Autodesk Fusion 360 part; units mm, degrees
box "BoxPrimitive1" add length 20.5 width 45.5 height 1.5 placed x (0, 1, 0) y (-1, 0, 0) z (0, 0, 1) at (45.5, 0, 0)
sketch "Sketch2" plane through (0, 0, 1.5) normal (0, 0, 1) x (-1, 0, 0)
  line L0 (-45.5, -20.5) -> (0, -20.5)
  line L1 (0, -20.5) -> (0, 0)
  line L2 (0, 0) -> (-45.5, 0)
  line L3 (-45.5, 0) -> (-45.5, -20.5)
  line L4 (-45.5, -20.5) -> (-35.75, -20.5)
  line L5 (-35.75, -20.5) -> (-35.75, -10.25)
  line L6 (0, -20.5) -> (-9.75, -20.5)
  line L7 (-9.75, -20.5) -> (-9.75, -10.25)
  dimension "d6" = 9.75
  dimension "d7" = 10.25
  dimension "d10" = 9.75
  dimension "d11" = 10.25
cylinder "CylinderPrimitive1" add diameter 16 height 12 placed x (1, 0, 0) y (0, 1, 0) z (0, 0, 1) at (35.75, 10.25, 1.5)
cylinder "CylinderPrimitive2" add diameter 16 height 12 placed x (1, 0, 0) y (0, 1, 0) z (0, 0, 1) at (9.75, 10.25, 1.5)
Can you work these out from the model? Positions are in its coordinate system, mm. A direction names the side the tool comes from. Coordinates: 2 decimals unless noted, no trailing zeros. Order: outer loops, then holes, each group sorted by start corner. A loop starts at its lowest first (then second) coordinate and runs counter-clockwise, first axis right, second up. Notation, with made-up numbers: M 47,53.25 L 73,53.25 A20 ccw 73,71.25 Z; hole C 18.25,58 d4. An arc over 180 degrees is marked long. Answer as CSV lines item,"result".
(1) Suppose I cut it at A-A on x = 35.75. Please give me the cut outline in (y, z).
Geometry check:
outline,"M 0,0 L 20.5,0 L 20.5,1.5 L 18.25,1.5 L 18.25,13.5 L 2.25,13.5 L 2.25,1.5 L 0,1.5 Z"
(2) Suppose I cut it at D-D on x = 14. Please give me the cut outline in (y, z), plus the area to 3 significant figures.
Geometry check:
outline,"M 0,0 L 20.5,0 L 20.5,1.5 L 17.03,1.5 L 17.03,13.5 L 3.47,13.5 L 3.47,1.5 L 0,1.5 Z"
area,"193 mm^2"
(3) Please list where these lines run through material, in increasing order: L1, parallel to Z at x = 41.5, y = 17; L2, parallel to X at y = 3, z = 10.5; L3, parallel to X at y = 10, z = 10.75.
Geometry check:
L1,"0 to 1.5"
L2,"6.37 to 13.13, 32.37 to 39.13"
L3,"1.75 to 17.75, 27.75 to 43.75"
(4) I'm going to push flat-ended pins straight in: pin 1 (5 mm diameter, centred on x = 38, z = 10.5, fed in from +Y); pin 2 (2 mm diameter, centred on x = 14.5, z = 4.5, fed in from +Y); pin 3 (3 mm diameter, centred on x = 25, y = 3, fed in from +Z). Where does each tip first touch, or does it pass through?
Geometry check:
pin 1,"y = 18.25"
pin 2,"y = 17.32"
pin 3,"z = 1.5"
(5) If we mould it in two halves opening along X, with no side actions, what happens to faces 3 (the flat face through (22, 10, 1.5)), 4 (the flat face through (45.5, 10, 1)), 5 (the flat face through (10, 10, 13.5)), 6 (the cylindrical face through (29.401, 5.382, 7.584))? For each: released by +X, released by -X, zero draft, split by the parting line, or undercut.
Geometry check:
face 3,"undercut"
face 4,"released by +X"
face 5,"zero draft"
face 6,"undercut"
(6) Suppose I cut it at B-B on y = 10.25. Please give me the cut outline in (x, z).
Geometry check:
outline,"M 0,0 L 45.5,0 L 45.5,1.5 L 43.75,1.5 L 43.75,13.5 L 27.75,13.5 L 27.75,1.5 L 17.75,1.5 L 17.75,13.5 L 1.75,13.5 L 1.75,1.5 L 0,1.5 Z"
(7) On a 3-axis mill with a long thin cutter (end or side, diameter ignored), from which of +Z, -Z, +X, -X, +Y, -Y can I reach the whole of each face in a straight line? I mean faces 1 (the flat face through (23, 20.5, 1)), 2 (the cylindrical face through (8.02, 2.44, 7.58)). Say none if no direction works.
Geometry check:
face 1,"+Z, -Z, +X, -X, +Y"
face 2,"+Z"
(8) Suppose I cut it at C-C on z = 12.5. Please give me the cut outline in (x, y).
Geometry check:
outline,"C 9.75,10.25 d16; C 35.75,10.25 d16"
